```python
from build123d import *

# Parameters (mm, degrees)
SKETCH1_R           = 30
BOSS_EXTRUDE1_DEPTH = 30
SKETCH2_R           = 15
CUT_EXTRUDE1_DEPTH  = 10
SKETCH3_R           = 5
CUT_EXTRUDE2_DEPTH  = 10
SKETCH5_R           = 5
CUT_EXTRUDE5_DEPTH  = 110
CUT_EXTRUDE6_DEPTH  = 20
SKETCH7_R           = 2.5
CUT_EXTRUDE7_DEPTH  = 20
SKETCH8_R           = 5
CUT_EXTRUDE8_DEPTH  = 10
SKETCH9_R           = 10
CUT_EXTRUDE9_DEPTH  = 10


with BuildPart() as part:
    # Sketch1 → Boss-Extrude1 (new body)
    with BuildSketch(Plane.XY):
        Circle(SKETCH1_R)
    extrude(amount=BOSS_EXTRUDE1_DEPTH)

    # Sketch2 → Cut-Extrude1 (cut)
    with BuildSketch(Plane.XY.offset(30)):
        Circle(SKETCH2_R)
    extrude(amount=-CUT_EXTRUDE1_DEPTH, mode=Mode.SUBTRACT)

    # Sketch3 → Cut-Extrude2 (cut)
    with BuildSketch(Plane.XY.offset(20)):
        Circle(SKETCH3_R)
    extrude(amount=-CUT_EXTRUDE2_DEPTH, mode=Mode.SUBTRACT)

    # Sketch5 → Cut-Extrude5 (cut)
    with BuildSketch(Plane.XY.offset(30)):
        with Locations((20, -10)):
            Circle(SKETCH5_R)
        with Locations((-20, -10)):
            Circle(SKETCH5_R)
    extrude(amount=-CUT_EXTRUDE5_DEPTH, mode=Mode.SUBTRACT)

    # Sketch6 → Cut-Extrude6 (cut)
    with BuildSketch(Plane.XY.offset(30)):
        with BuildLine():
            Line((-10, 28.284271247), (-10, 11.180339887))
            ThreePointArc((-10, 11.180339887), (0, 15), (10, 11.180339887))
            Line((10, 11.180339887), (10, 28.284271247))
            ThreePointArc((10, 28.284271247), (0, 30), (-10, 28.284271247))
        make_face()
    extrude(amount=-CUT_EXTRUDE6_DEPTH, mode=Mode.SUBTRACT)

    # Sketch7 → Cut-Extrude7 (cut)
    with BuildSketch(Plane.XY.offset(10)):
        with Locations((0, 22.5)):
            Circle(SKETCH7_R)
    extrude(amount=-CUT_EXTRUDE7_DEPTH, mode=Mode.SUBTRACT)

    # Sketch8 → Cut-Extrude8 (cut)
    with BuildSketch(Plane.XY.offset(10)):
        Circle(SKETCH8_R)
    extrude(amount=-CUT_EXTRUDE8_DEPTH, mode=Mode.SUBTRACT)

    # Sketch9 → Cut-Extrude9 (cut)
    with BuildSketch(Plane(origin=(0, 0, 0), x_dir=(-1, 0, 0), z_dir=(0, 0, -1))):
        Circle(SKETCH9_R)
    extrude(amount=-CUT_EXTRUDE9_DEPTH, mode=Mode.SUBTRACT)


solid = part.part
```
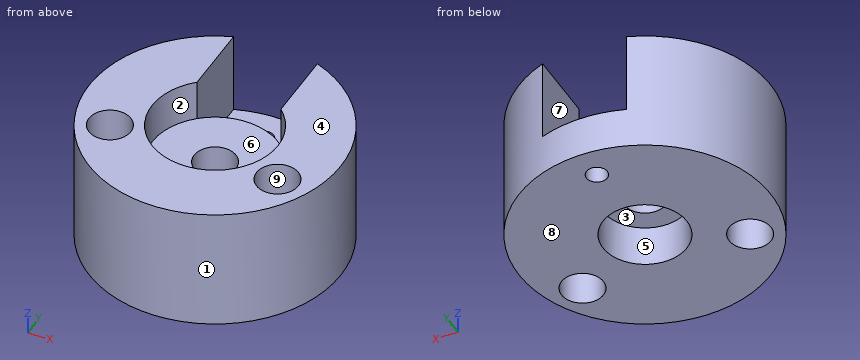
CAD build for the part. Positions are in the model's coordinates, mm. Face numbers are marked on the shaded views. A direction names the side the tool comes from. Coordinates: 2 decimals unless noted, no trailing zeros. Order: outer loops, then holes, each group sorted by start corner. A loop starts at its lowest first (then second) coordinate and runs counter-clockwise, first axis right, second up. Notation, with made-up numbers: (81.5, -40) - (107.5, -40) arc R16 cw to (107.5, -33) - close; hole circle Ø1 at (-12.75, 69). An arc over 180 degrees is marked (long way). Use a Markdown table: item, result. Add a question column.
(1) Saw through at D-D (x = -16). Give the cut face in (y, z), then the cut area to 3 significant figures.
(2) Which spindle directions (+Z, -Z, +X, -X, +Y, -Y) get a long thin tool onto all of the face, cutting with end or side? Do the marked faces 5, 6, 7, 8 and 9. Say none if no direction does.
(3) Drill centre lines: line 1 along Y through (x, z) = (0, 5.5); line 2 along Y through (x, z) = (0, 13.25); line 3 along X through (y, z) = (0, 24.5). Where is each one in solid material? Low to high. Write a range as [from, to].
(4) Saw through at C-C (z = 14.5). Give the cut face in (x, y).
(5) Pull direction X, two halves, no side cores. Call the marked faces 1, 2, 3 and 4: +X half, -X half, draft (parallel to the pull), parting line (faces both ways), or undercut.
(6) Saw through at A-A (x = 0). Give the cut face in (y, z).
(7) Saw through at B-B (y = 0). Give the cut face in (x, z), then the cut area to 3 significant figures.
(8) Flat gauge pins, fed straight in: pin 1 (1.5 mm diameter, centred on x = -14, z = 12, fed in from +Y); pin 2 (11.5 mm diameter, centred on x = 0, y = 0, fed in from -Z); pin 3 (6 mm diameter, centred on x = 0, y = 22.5, fed in from +Z); pin 4 (5 mm diameter, centred on x = -4, y = 20.5, fed in from -Z). Where does each tip first touch, or does it go through?
Solved:
| question | item | result |
|---|---|---|
| 1 | outline | (-25.38, 0) - (-13, 0) - (-13, 30) - (-25.38, 30) - close; (-7, 0) - (25.38, 0) - (25.38, 30) - (-7, 30) - close |
| 1 | area | 1,340 mm² |
| 2 | face 5 | -Z |
| 2 | face 6 | +Z |
| 2 | face 7 | +Z, +Y |
| 2 | face 8 | -Z, +X, -X, +Y, -Y |
| 2 | face 9 | +Z, -Z |
| 3 | line 1 | y = [-30, -10], [10, 20], [25, 30] |
| 3 | line 2 | y = [-30, -5], [5, 15] |
| 3 | line 3 | x = [-30, -15], [15, 30] |
| 4 | outline | (-10, 11.18) - (-10, 28.28) arc R30 ccw (long way) to (10, 28.28) - (10, 11.18) arc R15 ccw to start; hole circle Ø10 at (-20, -10); hole circle Ø10 at (0, 0); hole circle Ø10 at (20, -10) |
| 5 | face 1 | parting line |
| 5 | face 2 | undercut |
| 5 | face 3 | undercut |
| 5 | face 4 | draft |
| 6 | outline | (-30, 0) - (-10, 0) - (-10, 10) - (-5, 10) - (-5, 20) - (-15, 20) - (-15, 30) - (-30, 30) - close; (5, 10) - (10, 10) - (10, 0) - (20, 0) - (20, 10) - (15, 10) - (15, 20) - (5, 20) - close; (25, 0) - (30, 0) - (30, 10) - (25, 10) - close |
| 7 | outline | (-30, 0) - (-10, 0) - (-10, 10) - (-5, 10) - (-5, 20) - (-15, 20) - (-15, 30) - (-30, 30) - close; (5, 10) - (10, 10) - (10, 0) - (30, 0) - (30, 30) - (15, 30) - (15, 20) - (5, 20) - close |
| 7 | area | 1,200 mm² |
| 8 | pin 1 | stops at y = 26.92 |
| 8 | pin 2 | stops at z = 10 |
| 8 | pin 3 | stops at z = 10 |
| 8 | pin 4 | stops at z = 0 |
